Part model, mm, in its own coordinate system. Face numbers are marked on the shaded views. Give positions to 0.01 mm unless a question says otherwise; leave off trailing zeros. Order: outer loops, then holes, each group sorted by start corner. A loop starts at its lowest first (then second) coordinate and runs counter-clockwise, first axis right, second up. Notation, with made-up numbers: (44, -38) - (99, -38) arc R18 cw to (99, -5) - close; hole circle Ø8 at (69.25, 26.25). An arc over 180 degrees is marked (long way). One line per item, written item: value.
```python
from build123d import *

# Parameters (mm, degrees)
F0_R     = 15
F0_R_2   = 5
F0_R_3   = 2.5
F1_DEPTH = 7
F2_SIZE  = 0.5
F3_SIZE  = 0.5


with BuildPart() as f1:
    # F0 (on Front) → F1 (new body)
    with BuildSketch(Plane.XZ):
        Circle(F0_R)
        Circle(F0_R_2, mode=Mode.SUBTRACT)
        with Locations((10, 0)):
            Circle(F0_R_3, mode=Mode.SUBTRACT)
    extrude(amount=F1_DEPTH)

    # F2
    f2_edges = [f1.edges().sort_by_distance(p)[0] for p in [
        (-15, -7, 0),
    ]]
    chamfer(f2_edges, length=F2_SIZE)

    # F3
    f3_edges = [f1.edges().sort_by_distance(p)[0] for p in [
        (-15, 0, 0),
    ]]
    chamfer(f3_edges, length=F3_SIZE)


solid = f1.part
```
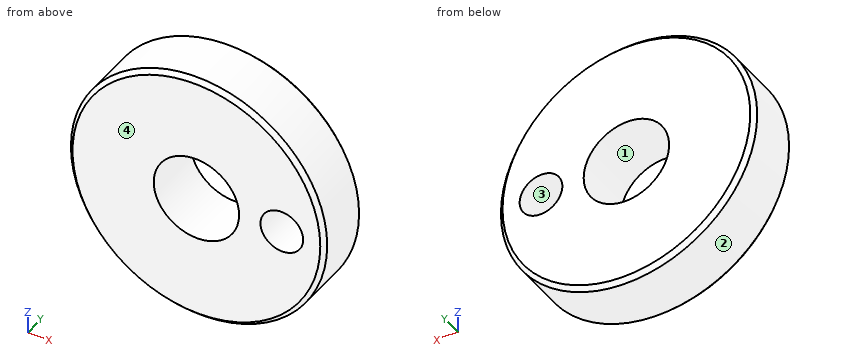
1) Cut at A-A, the plane x = 0. Give the cut face in (y, z).
Outcome:
outline: (-7, -14.5) - (-6.5, -15) - (-0.5, -15) - (0, -14.5) - (0, -5) - (-7, -5) - close; (-7, 5) - (0, 5) - (0, 14.5) - (-0.5, 15) - (-6.5, 15) - (-7, 14.5) - close
2) Cut at B-B, the plane z = 0. Give the cut face in (x, y), then the cut area to 4 significant figures.
Outcome:
outline: (-15, -6.5) - (-14.5, -7) - (-5, -7) - (-5, 0) - (-14.5, 0) - (-15, -0.5) - close; (5, -7) - (7.5, -7) - (7.5, 0) - (5, 0) - close; (12.5, -7) - (14.5, -7) - (15, -6.5) - (15, -0.5) - (14.5, 0) - (12.5, 0) - close
area: 104.5 mm^2
3) Drill centre lines: line 1 along Z through (x, y) = (0, -2.5); line 2 along Z through (x, y) = (-1.5, -4.25); line 3 along X through (y, z) = (-3, 8.75). Where is each one in solid material? Low to high. Write a range as from..to.
Outcome:
line 1: z = -15..-5, 5..15
line 2: z = -14.92..-4.77, 4.77..14.92
line 3: x = -12.18..12.18
4) Pin check, flat tips, straight feed: pin 1 (3 mm diameter, centred on y = -4.5, z = -4, fed in from -X); pin 2 (1.5 mm diameter, centred on x = -12, y = -5, fed in from +Z); pin 3 (4 mm diameter, centred on x = 10, y = -5, fed in from -Z). Stop position of each tip, or through.
Outcome:
pin 1: stops at x = -14.79
pin 2: stops at z = 9.92
pin 3: stops at z = -12.69
5) Cut at C-C, the plane y = -6. Give the cut face in (x, z).
Outcome:
outline: circle Ø30 at (0, 0); hole circle Ø10 at (0, 0); hole circle Ø5 at (10, 0)
6) Mould opens along Z. For the marked faces 1, 2, 3 and 4 say: released by +Z, released by -Z, zero draft, split by the parting line, or undercut.
Outcome:
face 1: undercut
face 2: split by the parting line
face 3: undercut
face 4: zero draft
